Could you check a few things on this model? Use its own coordinates, in mm. Coordinates: 2 decimals unless noted, no trailing zeros. Loops run counter-clockwise (first coordinate to the right, second up) from the corner with the lowest first, then second, coordinate; pieces in that order, holes last.
1) Imagine slicing it at A-A on x = -18.5. Please give me the cut outline in (y, z).
2) If I drill on line 1 along Y through (x, z) = (18.5, 9); line 2 along X through (y, z) = (-18, 9.3), over which ranges is the centre line in solid material (lowest first)?
3) Thinking about a two-plate mould opening in X: for faces 1 (the face through (0, 0, 8)), 2 (the face through (-32, 0, 9)), 3 (the face through (-18.708, 20.086, 8.789)), which applies, released by +X, released by -X, zero draft, split by the parting line, or undercut?
```python
from build123d import *

# Parameters (mm, degrees)
PCB_1_6_START         = 8
SKETCH_1_W            = 64
SKETCH_1_H            = 64
PCB_1_6_DEPTH         = 1.6
CUT_EXTRUDE_START     = 8
SKETCH_2_R            = 1.6
CUT_EXTRUDE_451_DEPTH = 1.6


with BuildPart() as part:
    # 草图1 → PCB外廓参考_板厚暂按1.6 (new body)
    with BuildSketch(Plane.XY.offset(PCB_1_6_START)):
        Rectangle(SKETCH_1_W, SKETCH_1_H)
    extrude(amount=PCB_1_6_DEPTH)

    # 草图2 → Cut-Extrude 451 (cut)
    with BuildSketch(Plane.XY.offset(CUT_EXTRUDE_START)):
        with Locations((-18.5, -18.5)):
            Circle(SKETCH_2_R)
        with Locations((-18.5, 18.5)):
            Circle(SKETCH_2_R)
        with Locations((18.5, -18.5)):
            Circle(SKETCH_2_R)
        with Locations((18.5, 18.5)):
            Circle(SKETCH_2_R)
    extrude(amount=CUT_EXTRUDE_451_DEPTH, mode=Mode.SUBTRACT)


solid = part.part
```
Filled in:
1. outline: (-32, 8) - (-20.1, 8) - (-20.1, 9.6) - (-32, 9.6) - close; (-16.9, 8) - (16.9, 8) - (16.9, 9.6) - (-16.9, 9.6) - close; (20.1, 8) - (32, 8) - (32, 9.6) - (20.1, 9.6) - close
2. line 1: y = -32 to -20.1, -16.9 to 16.9, 20.1 to 32
2. line 2: x = -32 to -20.02, -16.98 to 16.98, 20.02 to 32
3. face 1: zero draft
3. face 2: released by -X
3. face 3: undercut
